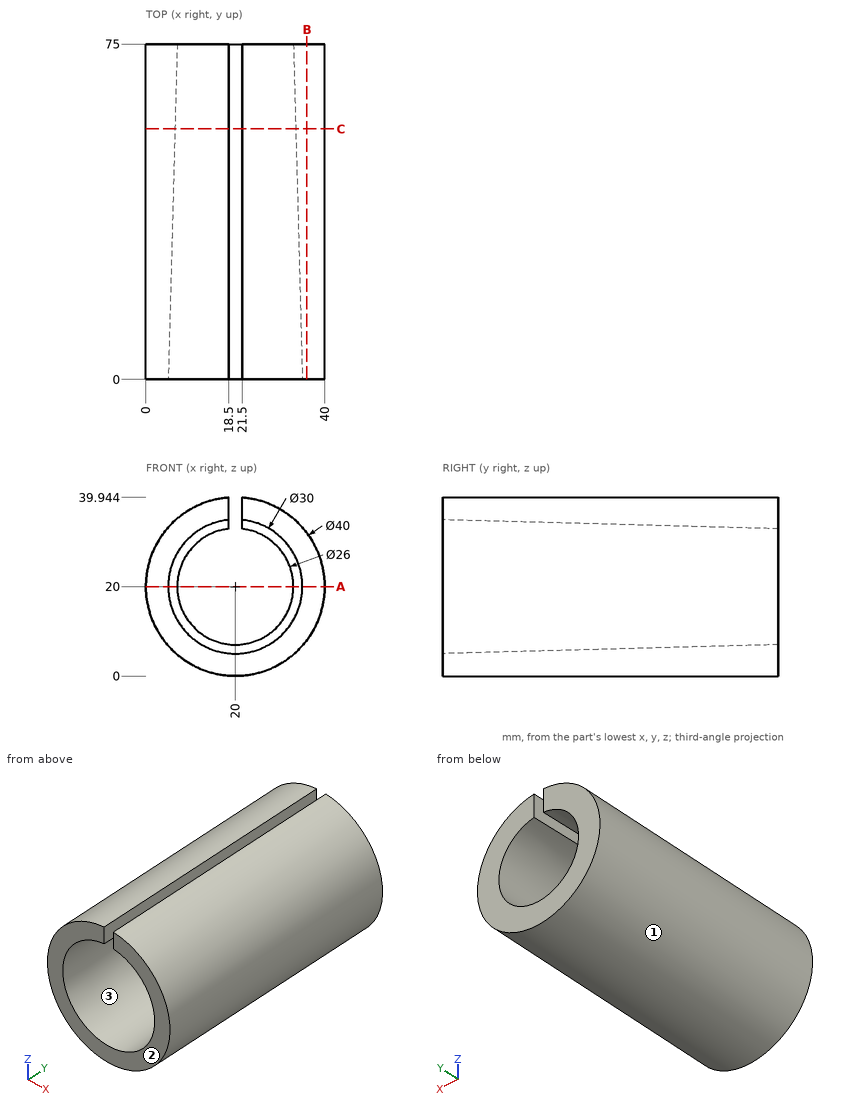
Study the drawing (mm; zero at the part's minimum x, y, z) and answer. Coordinates: 2 decimals unless noted, no trailing zeros. Loops run counter-clockwise (first coordinate to the right, second up) from the corner with the lowest first, then second, coordinate; pieces in that order, holes last. Notation, with made-up numbers: M 26,16 L 83,16 A16 cw 83,35 Z; hole C 36,-35 d9. An arc over 180 degrees is marked long. Answer in a Markdown table with one row per item.
1) Given pin 1 (3.5 mm diameter, centred on y = 48, z = 36, fed in from -X); pin 2 (6 mm diameter, centred on y = 41.5, z = 27, fed in from +X); pin 3 (3 mm diameter, centred on y = 44, z = 35.5, fed in from -X), each flat-ended and moving along its own axis, determine where each tip first touches the part or whether it passes through.
Answers below:
| item | result |
|---|---|
| pin 1 | x = 5.97 |
| pin 2 | x = 39.6 |
| pin 3 | x = 5.72 |
2) Find section C-C (y = 56). Determine the outline of the cut face in (x, z).
Answers below:
| item | result |
|---|---|
| outline | M 18.5,33.42 L 18.5,39.94 A20 ccw long 21.5,39.94 L 21.5,33.42 A13.51 cw long Z |
3) Determine the mould class of the marked faces 1, 2 and 3 for opening direction Z: released by +Z, released by -Z, zero draft, split by the parting line, or undercut.
Answers below:
| item | result |
|---|---|
| face 1 | split by the parting line |
| face 2 | zero draft |
| face 3 | undercut |
4) Find section B-B (x = 36). Determine the outline of the cut face in (y, z), then the cut area to 3 significant figures.
Answers below:
| item | result |
|---|---|
| outline | M 0,8 L 75,8 L 75,32 L 0,32 Z |
| area | 1,800 mm^2 |
5) Find the intervals of material crossed by probe 1 along X at (y, z) = (3, 31) (1 decimal); probe 2 along X at (y, z) = (49, 34.5) (1 decimal); probe 3 along Z at (x, y) = (15, 61.5) (1 decimal), in increasing order.
Answers below:
| item | result |
|---|---|
| probe 1 | 3.3 to 9.9, 30.1 to 36.7 |
| probe 2 | 6.2 to 18.5, 21.5 to 33.8 |
| probe 3 | 0.6 to 7.6, 32.4 to 39.4 |
6) Find section A-A (z = 20). Determine the outline of the cut face in (x, y).
Answers below:
| item | result |
|---|---|
| outline | M 0,0 L 5,0 L 7,75 L 0,75 Z; M 33,75 L 35,0 L 40,0 L 40,75 Z |
